Here's how the part is built. I have some questions about the finished solid (model axes, mm). Coordinates: 2 decimals unless noted, no trailing zeros. Order: outer loops, then holes, each group sorted by start corner. A loop starts at its lowest first (then second) coordinate and runs counter-clockwise, first axis right, second up. Notation, with made-up numbers: (80, -16.5) - (117, -16.5) arc R13 ccw to (117, -1.5) - close; hole circle Ø9 at (82, -30). An arc over 180 degrees is marked (long way). Answer as CSV lines item,"result". Start each with the question number.
Q1. For pin 1 Ø8 at (x, z) = (5, 30.5) entering from -Y, with a flat end and sliding along its axis, tell me the tip position at first contact or that it passes through.
Q2. Suppose I cut it at C-C (x = 32). Please give me the cut outline in (y, z).
Q3. Suppose I cut it at A-A (z = 18). Please give me the cut outline in (x, y), then the cut area to 3 significant figures.
Q4. Suppose I cut it at B-B (x = -56.8). Please give me the cut outline in (y, z).
Q5. Suppose I cut it at D-D (y = -1.1). Please give me the cut outline in (x, z).
Q6. I need wall thicknesses on line 1 (Z direction, x = 56.8, y = -2.1); line 2 (X direction, y = -0.05, z = 18.5); line 3 (Z direction, x = -56, y = -2.7). Which ranges of each line are inside material? Lowest first, please.
from build123d import *

# Parameters (mm, degrees)
F0_W     = 130
F0_H     = 80
F0_R     = 1.65
F0_W_2   = 105.7
F0_H_2   = 68.8
F1_DEPTH = 3


with BuildPart() as f1:
    # F0 (on Front) → F1 (new body)
    with BuildSketch(Plane.XZ):
        Rectangle(F0_W, F0_H)
        with Locations((-56.8, -33.85)):
            Circle(F0_R, mode=Mode.SUBTRACT)
        with Locations((56.8, -33.85)):
            Circle(F0_R, mode=Mode.SUBTRACT)
        with Locations((-56.8, 33.85)):
            Circle(F0_R, mode=Mode.SUBTRACT)
        Rectangle(F0_W_2, F0_H_2, mode=Mode.SUBTRACT)
        with Locations((56.8, 33.85)):
            Circle(F0_R, mode=Mode.SUBTRACT)
    extrude(amount=F1_DEPTH)


solid = f1.part
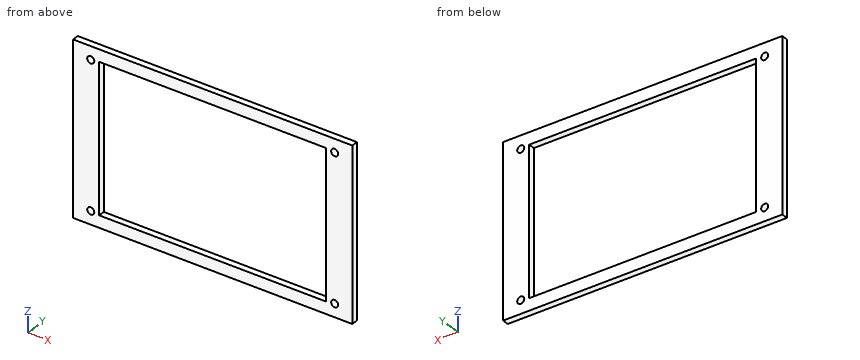
Here are the results:
1,pin 1,"stops at y = -3"
2,outline,"(-3, -40) - (0, -40) - (0, -34.4) - (-3, -34.4) - close; (-3, 34.4) - (0, 34.4) - (0, 40) - (-3, 40) - close"
3,outline,"(-65, -3) - (-52.85, -3) - (-52.85, 0) - (-65, 0) - close; (52.85, -3) - (65, -3) - (65, 0) - (52.85, 0) - close"
3,area,"72.9 mm²"
4,outline,"(-3, -40) - (0, -40) - (0, -35.5) - (-3, -35.5) - close; (-3, -32.2) - (0, -32.2) - (0, 32.2) - (-3, 32.2) - close; (-3, 35.5) - (0, 35.5) - (0, 40) - (-3, 40) - close"
5,outline,"(-65, -40) - (65, -40) - (65, 40) - (-65, 40) - close; hole circle Ø3.3 at (-56.8, -33.85); hole circle Ø3.3 at (-56.8, 33.85); hole (-52.85, -34.4) - (52.85, -34.4) - (52.85, 34.4) - (-52.85, 34.4) - close; hole circle Ø3.3 at (56.8, -33.85); hole circle Ø3.3 at (56.8, 33.85)"
6,line 1,"z = -40 to -35.5, -32.2 to 32.2, 35.5 to 40"
6,line 2,"x = -65 to -52.85, 52.85 to 65"
6,line 3,"z = -40 to -35.29, -32.41 to 32.41, 35.29 to 40"
